```python
from build123d import *

# Parameters (mm, degrees)
IZIM2_W                     = 6
IZIM2_H                     = 18
Y_KSEKLIK_EKSTR_ZYON1_DEPTH = 1.2
IZIM3_W                     = 6
IZIM3_H                     = 1.4
Y_KSEKLIK_EKSTR_ZYON4_DEPTH = 3.2
IZIM6_W                     = 6
IZIM6_H                     = 2
Y_KSEKLIK_EKSTR_ZYON5_DEPTH = 2
KES_EKSTR_ZYON2_DEPTH       = 6
IZIM8_W                     = 6
IZIM8_H                     = 2
Y_KSEKLIK_EKSTR_ZYON6_DEPTH = 2
KES_EKSTR_ZYON3_DEPTH       = 6
Y_KSEKLIK_EKSTR_ZYON8_DEPTH = 3.2
IZIM12_R                    = 0.75
KES_EKSTR_ZYON4_DEPTH       = 4


with BuildPart() as part:
    # Çizim2 → Yükseklik-Ekstrüzyon1 (new body)
    with BuildSketch(Plane.XY):
        Rectangle(IZIM2_W, IZIM2_H)
    extrude(amount=Y_KSEKLIK_EKSTR_ZYON1_DEPTH)

    # Çizim3 → Yükseklik-Ekstrüzyon4 (add)
    with BuildSketch(Plane.XY.offset(1.2)):
        with Locations((0, 8.3)):
            Rectangle(IZIM3_W, IZIM3_H)
        with Locations((0, -8.3)):
            Rectangle(IZIM3_W, IZIM3_H)
    extrude(amount=Y_KSEKLIK_EKSTR_ZYON4_DEPTH)

    # Çizim6 → Yükseklik-Ekstrüzyon5 (add)
    with BuildSketch(Plane.XY.offset(4.4)):
        with Locations((0, 8)):
            Rectangle(IZIM6_W, IZIM6_H)
    extrude(amount=Y_KSEKLIK_EKSTR_ZYON5_DEPTH)

    # Çizim7 → Kes-Ekstrüzyon2 (cut)
    with BuildSketch(Plane(origin=(3, 0, 0), x_dir=(0, 0, -1), z_dir=(1, 0, 0))):
        Polygon((-6.4, 9), (-4.4, 7), (-6.4, 7), align=None)
    extrude(amount=-KES_EKSTR_ZYON2_DEPTH, mode=Mode.SUBTRACT)

    # Çizim8 → Yükseklik-Ekstrüzyon6 (add)
    with BuildSketch(Plane.XY.offset(4.4)):
        with Locations((0, -8)):
            Rectangle(IZIM8_W, IZIM8_H)
    extrude(amount=Y_KSEKLIK_EKSTR_ZYON6_DEPTH)

    # Çizim9 → Kes-Ekstrüzyon3 (cut)
    with BuildSketch(Plane.ZY.offset(3)):
        Polygon((6.4, -9), (4.4, -7), (6.4, -7), align=None)
    extrude(amount=-KES_EKSTR_ZYON3_DEPTH, mode=Mode.SUBTRACT)

    # Çizim10 → Yükseklik-Ekstrüzyon8 (add)
    with BuildSketch(Plane(origin=(0, 0, 0), x_dir=(-1, 0, 0), z_dir=(0, 0, -1))):
        with BuildLine():
            Line((1.5, 1.5), (-1.5, 1.5))
            ThreePointArc((-1.5, 1.5), (-3, 0), (-1.5, -1.5))
            Line((-1.5, -1.5), (1.5, -1.5))
            ThreePointArc((1.5, -1.5), (3, 0), (1.5, 1.5))
        make_face()
    extrude(amount=Y_KSEKLIK_EKSTR_ZYON8_DEPTH)

    # Çizim12 → Kes-Ekstrüzyon4 (cut)
    with BuildSketch(Plane(origin=(0, 0, -3.2), x_dir=(-1, 0, 0), z_dir=(0, 0, -1))):
        Circle(IZIM12_R)
    extrude(amount=-KES_EKSTR_ZYON4_DEPTH, mode=Mode.SUBTRACT)


solid = part.part
```
Design review of the part built by this model. Coordinates are the model's own, in mm. A direction names the side the tool comes from. Coordinates: 2 decimals unless noted, no trailing zeros. Write each loop counter-clockwise with the first axis right and the second up, starting at its lowest first coordinate (ties: lowest second). Pieces come first, ordered by that corner, then holes. Notation, with made-up numbers: M 54,43.25 L 70,43.25 A18 cw 70,60.25 Z; hole C -2,52 d8. An arc over 180 degrees is marked long. Answer as a JSON object with one key per item and string values.
Item 1: Insertion check: pin 1 Ø3 at (x, y) = (-1.5, 7) entering from -Z; pin 2 Ø1.8 at (x, y) = (-1, 2) entering from +Z; pin 3 Ø2.5 at (x, z) = (-0.5, -2.5) entering from +Y. Each pin has a flat end and moves straight along its axis. Give the tip position at first contact, or say it passes through.
Outcome:
{"pin 1": "z = 0", "pin 2": "z = 1.2", "pin 3": "y = 1.5"}
Item 2: Draft analysis for pull direction X (two halves, no side actions). For faces 5 (the cylindrical face through (0.75, 0.03, -1.23)), 6 (the flat face through (0, -8, 5.4)), 7 (the flat face through (0, 0, 0.8)), 8 (the cylindrical face through (-3, 0, -2)), state which applies: pulls with the +X half, pulls with the -X half, needs draft (parallel to the pull), parting line crosses it, or undercut.
Outcome:
{"face 5": "undercut", "face 6": "needs draft", "face 7": "undercut", "face 8": "pulls with the -X half"}
Item 3: Add section B-B, the plane x = 0. Give the boundary of the cut face in (y, z).
Outcome:
{"outline": "M -9,0 L -1.5,0 L -1.5,-3.2 L -0.75,-3.2 L -0.75,0.8 L 0.75,0.8 L 0.75,-3.2 L 1.5,-3.2 L 1.5,0 L 9,0 L 9,6.4 L 7,4.4 L 7.6,4.4 L 7.6,1.2 L -7.6,1.2 L -7.6,4.4 L -7,4.4 L -9,6.4 Z"}
Item 4: Add section A-A, the plane z = 2.5. Give the boundary of the cut face in (x, y), and give its area (3 significant figures).
Outcome:
{"outline": "M -3,-9 L 3,-9 L 3,-7.6 L -3,-7.6 Z; M -3,7.6 L 3,7.6 L 3,9 L -3,9 Z", "area": "16.8 mm²"}
Item 5: Add section C-C, the plane z = -1. Give the boundary of the cut face in (x, y), and give its area (3 significant figures).
Outcome:
{"outline": "M -1.5,-1.5 L 1.5,-1.5 A1.5 ccw 1.5,1.5 L -1.5,1.5 A1.5 ccw Z; hole C 0,0 d1.5", "area": "14.3 mm²"}
Item 6: Add section D-D, the plane y = 6. Give the boundary of the cut face in (x, z), and give its area (3 significant figures).
Outcome:
{"outline": "M -3,0 L 3,0 L 3,1.2 L -3,1.2 Z", "area": "7.20 mm²"}
Item 7: Wall thickness on probe 1 along Y at (x, z) = (0, -0.9); probe 2 along Y at (x, z) = (0.6, 3.75); probe 3 along Z at (x, y) = (0.35, -4): over which ranges is each line inside the solid? List them lowest first.
Outcome:
{"probe 1": "-1.5 to -0.75, 0.75 to 1.5", "probe 2": "-9 to -7.6, 7.6 to 9", "probe 3": "0 to 1.2"}
Item 8: Machinability: for faces 1 (the flat face through (0, -1.5, -2)), 2 (the flat face through (0, 8, 5.4)), 3 (the cylindrical face through (3, 0, -2)), 4 (the flat face through (0, 1.5, -2)), which of the approach directions +Z, -Z, +X, -X, +Y, -Y give a long, thin tool a straight path to every point of the face, cutting with its end or side? Answer none if there is none.
Outcome:
{"face 1": "-Z, +X, -X, -Y", "face 2": "+Z, +X, -X", "face 3": "-Z, +X", "face 4": "-Z, +X, -X, +Y"}
